from build123d import *

# Parameters (mm, degrees)
CUT_EXTRUDE1_DEPTH  = 2.2225
SKETCH3_R           = 3.96875
BOSS_EXTRUDE1_DEPTH = 19.05
CHAMFER1_SIZE       = 1.27
CHAMFER1_SIZE2      = 0.733234842


with BuildPart() as part:
    # Sketch1 → Revolve1 (revolve)
    with BuildSketch(Plane(origin=(0, 0, 0), x_dir=(1, 0, 0), z_dir=(0, 1, 0))):
        with BuildLine():
            Line((6.946899945, -4.2164), (6.946899945, -3.689349932))
            ThreePointArc((6.946899945, -3.689349932), (5.758127461, -1.59917681), (3.962399967, 0))
            Line((3.962399967, 0), (-2.8e-08, 0))
            Line((-2.8e-08, 0), (-2.8e-08, -4.2164))
            Line((-2.8e-08, -4.2164), (6.946899945, -4.2164))
        make_face()
    revolve(axis=Axis((-2.8e-08, 0, 0), (0, 0, -1)))

    # Sketch2 → Cut-Extrude1 (cut)
    with BuildSketch(Plane(origin=(0, 0, 0), x_dir=(-1, 0, 0), z_dir=(0, 0, -1))):
        Polygon((2.749630657, 0), (1.374815329, 2.38125), (-1.374815329, 2.38125), (-2.749630657, 0), (-1.374815329, -2.38125), (1.374815329, -2.38125), align=None)
    extrude(amount=-CUT_EXTRUDE1_DEPTH, mode=Mode.SUBTRACT)

    # Sketch3 → Boss-Extrude1 (add)
    with BuildSketch(Plane.XY.offset(4.2164)):
        with Locations(Location((0, 0, 0), (0, 0, 180))):
            Circle(SKETCH3_R)
    extrude(amount=BOSS_EXTRUDE1_DEPTH)

    # Chamfer1
    chamfer1_edges = [part.edges().sort_by_distance(p)[0] for p in [
        (3.96875, 0, 23.2664),
    ]]
    chamfer1_side = [part.faces().sort_by_distance(p)[0] for p in [
        (3.96875, 0, 13.7414),
    ]]
    chamfer(chamfer1_edges, length=CHAMFER1_SIZE, length2=CHAMFER1_SIZE2, reference=chamfer1_side[0])


solid = part.part
Geometry: final body of the model. Coordinates: model frame, mm. A direction names the side the tool comes from. Coordinates: 2 decimals unless noted, no trailing zeros. Order: outer loops, then holes, each group sorted by start corner. A loop starts at its lowest first (then second) coordinate and runs counter-clockwise, first axis right, second up. Notation, with made-up numbers: (-37.5, 31) - (-28.5, 31) arc R25 cw to (-28.5, 52) - close; hole circle Ø10 at (-16, -32.75). An arc over 180 degrees is marked (long way). Use one line per item in the form item = value.
1) Pin query (flat end, axial travel): pin 1 (5 mm diameter, centred on x = -4.5, z = 17.5, fed in from +Y); pin 2 (6 mm diameter, centred on x = -5.5, z = 17.5, fed in from -Y); pin 3 (1.4 mm diameter, centred on x = 0, y = 0.5, fed in from -Z); pin 4 (4 mm diameter, centred on x = 1.5, z = 5.5, fed in from +Y). Return the tip coordinate at first contact, or that it passes through.
Solutions:
pin_1 = 3.43
pin_2 = -3.08
pin_3 = 2.22
pin_4 = 6.95
2) Section B-B (y = 6). Return loops of the section in (x, z).
Solutions:
outline = (-3.5, 3.69) arc R4.34 ccw to (3.5, 3.69) - (3.5, 4.22) - (-3.5, 4.22) - close
3) Mould query, pull axis X, two halves, no side actions, for faces 3 (the face through (-3, 3, 4.216)), 4 (the face through (0.86, 3.874, 12.982)), 5 (the face through (-2.072, 1.174, 1.096)). Classes: +X half, -X half, draft (parallel to the pull), parting line (faces both ways), or undercut.
Solutions:
face_3 = draft
face_4 = parting line
face_5 = undercut
4) Section A-A (x = 0). Return loops of the section in (y, z).
Solutions:
outline = (-6.95, 3.69) arc R7.41 ccw to (-3.96, 0) - (-2.38, 0) - (-2.38, 2.22) - (2.38, 2.22) - (2.38, 0) - (3.96, 0) arc R7.41 ccw to (6.95, 3.69) - (6.95, 4.22) - (3.97, 4.22) - (3.97, 22) - (3.24, 23.27) - (-3.24, 23.27) - (-3.97, 22) - (-3.97, 4.22) - (-6.95, 4.22) - close
5) Ray query, L1, parallel to Z at x = -0.25, y = 0.75; L2, parallel to Y at x = 0, z = 20.5; L3, parallel to Y at x = -2, z = 8. Return the intervals inside material, ascending.
Solutions:
L1 = 2.22 to 23.27
L2 = -3.97 to 3.97
L3 = -3.43 to 3.43
6) Section D-D (x = 5.25). Return loops of the section in (y, z), then the cut area to 3 significant figures.
Solutions:
outline = (-4.55, 3.69) arc R5.22 ccw to (4.55, 3.69) - (4.55, 4.22) - (-4.55, 4.22) - close
area = 22.0 mm^2
7) Section C-C (z = 22.25). Return loops of the section in (x, y).
Solutions:
outline = circle Ø7.64 at (0, 0)
8) Set-up query: faces 1 (the face through (2, -2, 0)), 2 (the face through (-2.05, -1.21, 1.1)). Return all of +Z, -Z, +X, -X, +Y, -Y with unobstructed straight access to the full face (end or side cutting, diameter ignored); none if empty.
Solutions:
face_1 = -Z, +X, -X, +Y, -Y
face_2 = -Z
